Read the model definition and answer for the solid it produces. Units are mm, in the model's axes. A direction names the side the tool comes from. Coordinates: 2 decimals unless noted, no trailing zeros. Write each loop counter-clockwise with the first axis right and the second up, starting at its lowest first coordinate (ties: lowest second). Pieces come first, ordered by that corner, then holes.
Item 1: Each of these flat-tipped pins is pushed along its axis until it touches: P1, Ø3, axis at x = -16, z = 6, coming from the +Y side; P2, Ø5, axis at x = -6.5, z = 13, coming from the +Y side; P3, Ø1, axis at y = -17.5, z = 21, coming from the -X side; P4, Ø1.5, axis at y = -21.5, z = 23, coming from the -X side. Where does it stop, or does it pass through?
Item 2: Section C-C (z = 8) is taken. Give the vertices of the cut face in (x, y), then the cut area to 3 significant figures.
Item 3: Section A-A (y = 0) is taken. Give the vertices of the cut face in (x, z).
Item 4: A tool of negligible diameter and unlimited length cuts with its end or side. For faces 1 (the face through (-4.336, -19.524, 19.818)), 2 (the face through (0, 0, 35)), from which of +Z, -Z, +X, -X, +Y, -Y can it reach the whole face along a straight path? Write none if from no direction.
Item 5: Straight lines are drawn through the part: probe 1 along Z at (x, y) = (17.5, 15); probe 2 along X at (y, z) = (-11, 4); probe 3 along Z at (x, y) = (12, -15.5). For each, find the intervals that lie inside material, in ascending order.
from build123d import *

# Parameters (mm, degrees)
F0_R     = 31
F1_DEPTH = 5
F2_R     = 20
F3_DEPTH = 30
F4_R     = 2


with BuildPart() as f1:
    # F0 (on Top) → F1 (new body)
    with BuildSketch(Plane.XY):
        Circle(F0_R)
    extrude(amount=F1_DEPTH)

    # F2 (on face) → F3 (join)
    with BuildSketch(Plane.XY.offset(5)):
        Circle(F2_R)
    extrude(amount=F3_DEPTH)

    # F4
    f4_edges = [f1.edges().sort_by_distance(p)[0] for p in [
        (-20, 0, 35),
        (-20, 0, 5),
        (-31, 0, 0),
    ]]
    fillet(f4_edges, radius=F4_R)


solid = f1.part
Established:
1. P1: stops at y = 27.19
1. P2: stops at y = 19.6
1. P3: stops at x = -10.54
1. P4: passes through
2. outline: circle Ø40 at (0, 0)
2. area: 1,260 mm2
3. outline: (-31, 2) arc R2 ccw to (-29, 0) - (29, 0) arc R2 ccw to (31, 2) - (31, 5) - (22, 5) arc R2 cw to (20, 7) - (20, 33) arc R2 ccw to (18, 35) - (-18, 35) arc R2 ccw to (-20, 33) - (-20, 7) arc R2 cw to (-22, 5) - (-31, 5) - close
4. face 1: +Z
4. face 2: +Z, +X, -X, +Y, -Y
5. probe 1: z = 0 to 5
5. probe 2: x = -28.98 to 28.98
5. probe 3: z = 0 to 34.2
